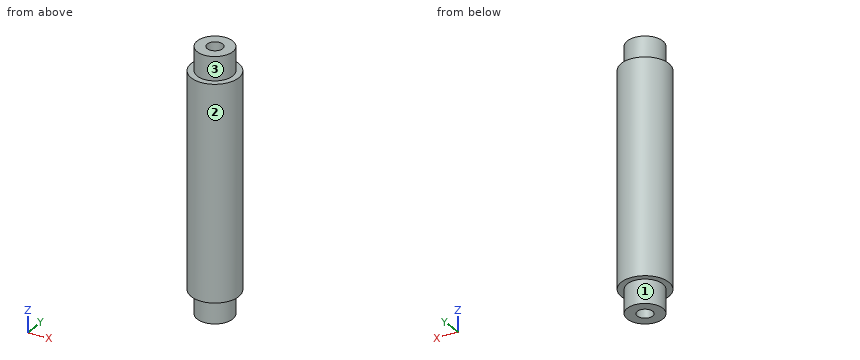
Autodesk Inventor part; units mm, degrees
ref_plane "Work Plane4" through (0, 0, -12.7) normal (0, 0, 1) x (1, 0, 0)
ref_plane "Work Plane5" through (0, 0, -69.85) normal (0, 0, -1) x (-1, 0, 0)
ref_plane "YZ Plane" through (0, 0, 0) normal (1, 0, 0) x (0, 1, 0)
sketch "Sketch1" plane through (0, 0, 0) normal (0, 0, 1) x (1, 0, 0)
  circle A0 centre (0, 0) radius 6.35
  dimension "d0" = 12.7
extrude "Extrusion1" add sketch "Sketch1" against normal blind 82.55
ref_plane "Work Plane4" through (0, 0, -12.7) normal (0, 0, 1) x (1, 0, 0)
sketch "Sketch4" plane through (0, 0, -12.7) normal (0, 0, 1) x (1, 0, 0)
  circle A0 centre (0, 0) radius 6.35
  circle A1 centre (0, 0) radius 4.7625
  circle A2 centre (0, 0) radius 1.7272
  dimension "d27" = 9.525
  dimension "d36" = 3.4544
ref_plane "Work Plane5" through (0, 0, -69.85) normal (0, 0, -1) x (-1, 0, 0)
sketch "Sketch5" plane through (0, 0, -69.85) normal (0, 0, -1) x (-1, 0, 0)
  circle A0 centre (0, 0) radius 6.35
  circle A1 centre (0, 0) radius 4.7625
  circle A2 centre (0, 0) radius 2.0828
  dimension "d24" = 9.525
  dimension "d35" = 4.1656
extrude "Extrusion6" cut sketch "Sketch5" along normal blind 25.4 contours A0 | A1 | A2
extrude "Extrusion7" cut sketch "Sketch4" along normal blind 25.4 contours A0 | A1 | A2
extrude "Extrusion8" add sketch "Sketch4" along normal blind 6.35 contours A1 | A2
extrude "Extrusion9" add sketch "Sketch5" along normal blind 6.35 contours A1 | A2
extrude "Extrusion10" cut sketch "Sketch5" along normal through all both and the other way through all contours A2
thread "Thread6"
properties part number "lower box weel shaft steel"
Geometry: final body of the model. Coordinates: model frame, mm. Face numbers are marked on the shaded views. A direction names the side the tool comes from. Coordinates: 2 decimals unless noted, no trailing zeros. Loops run counter-clockwise (first coordinate to the right, second up) from the corner with the lowest first, then second, coordinate; pieces in that order, holes last. Notation, with made-up numbers: (-17, -32.75) -> (21, -32.75) arc R31 ccw to (21, 3.25) -> close; hole circle Ø7 at (19, -10.5). An arc over 180 degrees is marked (long way). Use a Markdown table: item, result. Add a question column.
(1) Pin query (flat end, axial travel): pin 1 Ø2 at (x, z) = (-2, -39) entering from +Y; pin 2 Ø5 at (y, z) = (-5, -24) entering from -X; pin 3 Ø3 at (y, z) = (-2.5, -32.5) entering from -X. Return the tip coordinate at first contact, or that it passes through.
(2) Section query C-C, the plane z = -33. Return loops of the section in (x, y).
(3) Access query for the marked faces 1, 2 and 3. Directions: +Z, -Z, +X, -X, +Y, -Y. A direction counts if a zero-diameter tool reaches every point of the face in a straight line with its end or side. Return the directions, or none.
(4) Section query A-A, the plane x = 0. Return loops of the section in (y, z), plus the area to 3 significant figures.
(5) Section query D-D, the plane y = -4. Return loops of the section in (x, z), plus the area to 3 significant figures.
(6) Line query: line 1 along Y through (x, z) = (0, -57); line 2 along Z through (x, y) = (4.75, 3.25); line 3 along X through (y, z) = (-1.5, -34.5). Output: solid intervals per line, ascending.
Answer:
| question | item | result |
|---|---|---|
| 1 | pin 1 | stops at y = 6.27 |
| 1 | pin 2 | stops at x = -5.84 |
| 1 | pin 3 | stops at x = -6.27 |
| 2 | outline | circle Ø12.7 at (0, 0); hole circle Ø4.17 at (0, 0) |
| 3 | face 1 | -Z |
| 3 | face 2 | +Z, -Z |
| 3 | face 3 | +Z |
| 4 | outline | (-6.35, -69.85) -> (-4.76, -69.85) -> (-4.76, -76.2) -> (-2.08, -76.2) -> (-2.08, -6.35) -> (-4.76, -6.35) -> (-4.76, -12.7) -> (-6.35, -12.7) -> close; (2.08, -76.2) -> (4.76, -76.2) -> (4.76, -69.85) -> (6.35, -69.85) -> (6.35, -12.7) -> (4.76, -12.7) -> (4.76, -6.35) -> (2.08, -6.35) -> close |
| 4 | area | 556 mm^2 |
| 5 | outline | (-4.93, -69.85) -> (-2.58, -69.85) -> (-2.58, -76.2) -> (2.58, -76.2) -> (2.58, -69.85) -> (4.93, -69.85) -> (4.93, -12.7) -> (2.58, -12.7) -> (2.58, -6.35) -> (-2.58, -6.35) -> (-2.58, -12.7) -> (-4.93, -12.7) -> close |
| 5 | area | 629 mm^2 |
| 6 | line 1 | y = -6.35 to -2.08, 2.08 to 6.35 |
| 6 | line 2 | z = -69.85 to -12.7 |
| 6 | line 3 | x = -6.17 to -1.45, 1.45 to 6.17 |
